from build123d import *

# Parameters (mm, degrees)
SKETCH2_R               = 13.97
BOSS_EXTRUDE1_DEPTH     = 38.1
CHAMFER1_SIZE           = 5.08
SKETCH4_R               = 6.35
CUT_EXTRUDE1_DEPTH      = 127
SKETCH5_R               = 7.9375
CUT_EXTRUDE2_DEPTH      = 1.27
CUT_EXTRUDE3_START      = -1.27
SKETCH6_R               = 7.9375
CUT_EXTRUDE3_DEPTH      = 1.27
SKETCH8_W               = 3.81
SKETCH8_H               = 23.495
CUT_EXTRUDE4_DEPTH      = 12.7
SKETCH9_W               = 12.7
SKETCH9_H               = 0.508
CUT_EXTRUDE5_DEPTH      = 9.525
SKETCH10_R              = 1.5875
CUT_EXTRUDE6_DEPTH      = 2.54
SKETCH11_R              = 3.175
CUT_EXTRUDE7_DEPTH      = 6.35
SKETCH12_R              = 3.0226
CUT_EXTRUDE8_DEPTH      = 4.064
CIRPATTERN1_COUNT       = 4
CUT_EXTRUDE9_REACH      = 47.27
CUT_EXTRUDE9_END_RADIUS = 6.35
SKETCH13_R              = 1.27
CIRPATTERN2_START       = -6.096
CIRPATTERN2_OUTLINE_R   = 1.27
CIRPATTERN2_DEPTH       = 6.096
CHAMFER2_SIZE           = 0.254


with BuildPart() as part:
    # Sketch2 → Boss-Extrude1 (new body)
    with BuildSketch(Plane(origin=(0, 0, 0), x_dir=(1, 0, 0), z_dir=(0, 1, 0))):
        with Locations(Location((0, 0, 0), (0, 0, 90))):
            Circle(SKETCH2_R)
    extrude(amount=BOSS_EXTRUDE1_DEPTH)

    # Chamfer1
    chamfer1_edges = [part.edges().sort_by_distance(p)[0] for p in [
        (0, 38.1, 13.97),
    ]]
    chamfer(chamfer1_edges, length=CHAMFER1_SIZE)

    # Sketch4 → Cut-Extrude1 (cut)
    with BuildSketch(Plane.XZ):
        with Locations(Location((0, 0, 0), (0, 0, 270))):
            Circle(SKETCH4_R)
    extrude(amount=-CUT_EXTRUDE1_DEPTH, mode=Mode.SUBTRACT)

    # Sketch5 → Cut-Extrude2 (cut)
    with BuildSketch(Plane(origin=(0, 38.1, 0), x_dir=(1, 0, 0), z_dir=(0, 1, 0))):
        with Locations(Location((0, 0, 0), (0, 0, 270))):
            Circle(SKETCH5_R)
    extrude(amount=-CUT_EXTRUDE2_DEPTH, mode=Mode.SUBTRACT)

    # Sketch6 → Cut-Extrude3 (cut)
    with BuildSketch(Plane.XZ.offset(CUT_EXTRUDE3_START)):
        with Locations(Location((0, 0, 0), (0, 0, 90))):
            Circle(SKETCH6_R)
    extrude(amount=CUT_EXTRUDE3_DEPTH, mode=Mode.SUBTRACT)

    # Sketch8 → Cut-Extrude4 (cut, symmetric)
    with BuildSketch(Plane(origin=(0, 0, 0), x_dir=(0, 0, -1), z_dir=(1, 0, 0))):
        with Locations((12.065, 19.1135)):
            Rectangle(SKETCH8_W, SKETCH8_H)
    extrude(amount=CUT_EXTRUDE4_DEPTH, both=True, mode=Mode.SUBTRACT)

    # Sketch9 → Cut-Extrude5 (cut, symmetric)
    with BuildSketch(Plane(origin=(0, 0, 0), x_dir=(1, 0, 0), z_dir=(0, 1, 0))):
        with Locations((0, 13.97)):
            Rectangle(SKETCH9_W, SKETCH9_H)
    extrude(amount=CUT_EXTRUDE5_DEPTH, both=True, mode=Mode.SUBTRACT)

    # Sketch10 → Cut-Extrude6 (cut, symmetric)
    with BuildSketch(Plane(origin=(0, 0, -13.716), x_dir=(-1, 0, 0), z_dir=(0, 0, -1))):
        with Locations((0, 3.683)):
            Circle(SKETCH10_R)
    extrude(amount=CUT_EXTRUDE6_DEPTH, both=True, mode=Mode.SUBTRACT)

    # Sketch11 → Cut-Extrude7 (cut, symmetric)
    with BuildSketch(Plane(origin=(0, 0, -10.16), x_dir=(-1, 0, 0), z_dir=(0, 0, -1))):
        with Locations(Location((0, 19.1135, 0), (0, 0, 270))):
            Circle(SKETCH11_R)
    extrude(amount=CUT_EXTRUDE7_DEPTH, both=True, mode=Mode.SUBTRACT)

    # Sketch12 → Cut-Extrude8 (cut)
    with BuildSketch(Plane(origin=(0, 0, -10.16), x_dir=(-1, 0, 0), z_dir=(0, 0, -1))):
        with Locations(Location((4.939140867, 24.052640867, 0), (0, 0, 90))):
            Circle(SKETCH12_R)
    cut_extrude8 = extrude(amount=-CUT_EXTRUDE8_DEPTH, mode=Mode.SUBTRACT)

    # CirPattern1: Cut-Extrude8 ×4 about axis
    cirpattern1_axis = Axis((0, 19.1135, 0), (0, 0, 1))
    for i in range(1, CIRPATTERN1_COUNT):
        add(cut_extrude8.rotate(cirpattern1_axis, i * 360 / CIRPATTERN1_COUNT), mode=Mode.SUBTRACT)

    # Cut-Extrude9: up to this cylinder (the profile starts outside it)
    cut_extrude9_end = Plane(origin=(0, 14.174359, 0), z_dir=(0, -1, 0)) * Cylinder(CUT_EXTRUDE9_END_RADIUS, 108.24, mode=Mode.PRIVATE)
    # Sketch13 → Cut-Extrude9 (cut, up to the surface)
    with BuildSketch(Plane(origin=(0, 0, -6.096), x_dir=(-1, 0, 0), z_dir=(0, 0, -1)), mode=Mode.PRIVATE) as cut_extrude9_sk1:
        with Locations((4.939140867, 14.174359133)):
            Circle(SKETCH13_R)
    cut_extrude9_tool1 = extrude(cut_extrude9_sk1.sketch, amount=-CUT_EXTRUDE9_REACH, mode=Mode.PRIVATE) - cut_extrude9_end
    add(cut_extrude9_tool1.solids().sort_by_distance((-4.939141, 14.174359, -6.096))[0], mode=Mode.SUBTRACT)

    # CirPattern2: read off the stored shape, not the designer's step
    # CirPattern2 outline → CirPattern2 (cut)
    with BuildSketch(Plane.XY.offset(CIRPATTERN2_START)):
        with Locations((-4.939140867, 24.052640867)):
            Circle(CIRPATTERN2_OUTLINE_R)
        with Locations((4.939140867, 24.052640867)):
            Circle(CIRPATTERN2_OUTLINE_R)
        with Locations((4.939140867, 14.174359133)):
            Circle(CIRPATTERN2_OUTLINE_R)
    extrude(amount=CIRPATTERN2_DEPTH, mode=Mode.SUBTRACT)

    # Chamfer2
    chamfer2_edges = [part.edges().sort_by_distance(p)[0] for p in [
        (0, 38.1, -7.9375),
        (0, 0, -7.9375),
        (0, 0, 13.97),
        (0, 0, -13.716),
        (1.5875, 3.683, -13.716),
        (0, 22.2885, -10.16),
        (-4.939140867, 21.030040867, -10.16),
        (-1.916540867, 14.174359133, -10.16),
        (4.939140867, 17.196959133, -10.16),
        (1.916540867, 24.052640867, -10.16),
    ]]
    chamfer(chamfer2_edges, length=CHAMFER2_SIZE - 0.0001)  # a hair under: the kernel refuses the full size


solid = part.part
Geometry: final body of the model. Coordinates: model frame, mm. A direction names the side the tool comes from. Coordinates: 2 decimals unless noted, no trailing zeros. Loops run counter-clockwise (first coordinate to the right, second up) from the corner with the lowest first, then second, coordinate; pieces in that order, holes last. Notation, with made-up numbers: M -5.75,-9 L 29.25,-9 A26 ccw 29.25,11 Z; hole C 15.5,18.5 d4. An arc over 180 degrees is marked long. One line per item, written item: value. Start each with the question number.
1) Cut plane B-B (x = 0). Count the separate pieces of the cut face and the enclosed holes in it, then the cut area to 3 significant figures.
2) Cut plane C-C (y = 9.5). Return loops of the section in (x, z).
3) Cut plane A-A (z = 0). Return loops of the section in (x, y), then the cut area to 3 significant figures.
4) Draft query along Y for faces 1 (the flat face through (6, 0, -6)), 2 (the flat face through (2, 16, -10.16)), 3 (the flat face through (3, 38.1, -8)). Return one class per face: released by +Y, released by -Y, zero draft, split by the parting line, or undercut.
5) Material intervals for L1, parallel to Y at x = -6, z = -7; L2, parallel to X at y = 28, z = 0.25; L3, parallel to Y at x = -5.25, z = 5.75, sorted ascending. Write a range as from..to.
6) Reachability of faces 4 (the flat face through (7, 36.83, 0)), 5 (the cylindrical face through (6.78, 16.57, -8.03)), 6 (the cylindrical face through (7.75, 0.77, -1.72)), 7 (the cylindrical face through (0.279, 18.801, 6.344)) from +Z, -Z, +X, -X, +Y, -Y: full face, straight path, thin tool, end or side. Return the list, or none.
7) Pin query (flat end, axial travel): P1, Ø1, axis at y = 8, z = 11, coming from the +X side; P2, Ø1.5, axis at y = 23.5, z = 5.5, coming from the +X side; P3, Ø2, axis at x = -5, y = 34, coming from the -Z side. Return the tip coordinate at first contact, or that it passes through.
Evaluation:
1. separate pieces: 3
1. enclosed holes: 0
1. area: 423 mm^2
2. outline: M -9.59,-10.16 L 9.59,-10.16 A13.97 ccw long Z; hole C 0,0 d12.7
3. outline: M -13.97,0.25 L -13.72,0 L -8.19,0 L -7.94,0.25 L -7.94,1.27 L -6.35,1.27 L -6.35,36.83 L -7.94,36.83 L -7.94,37.85 L -8.19,38.1 L -8.89,38.1 L -13.97,33.02 Z; M 6.35,1.27 L 7.94,1.27 L 7.94,0.25 L 8.19,0 L 13.72,0 L 13.97,0.25 L 13.97,33.02 L 8.89,38.1 L 8.19,38.1 L 7.94,37.85 L 7.94,36.83 L 6.35,36.83 Z
3. area: 547 mm^2
4. face 1: released by -Y
4. face 2: undercut
4. face 3: released by +Y
5. L1: 0..11.34, 17..21.22, 26.88..37.77
5. L2: -13.97..-6.35, 6.35..13.97
5. L3: 1.27..36.83
6. face 4: +Y
6. face 5: -Z
6. face 6: -Y
6. face 7: +Y, -Y
7. P1: x = 9.21
7. P2: x = 13.14
7. P3: z = -13.13
